Could you check a few things on this model? Use its own coordinates, in mm. Face numbers are marked on the shaded views. A direction names the side the tool comes from. Coordinates: 2 decimals unless noted, no trailing zeros. Order: outer loops, then holes, each group sorted by start corner. A loop starts at its lowest first (then second) coordinate and runs counter-clockwise, first axis right, second up. Notation, with made-up numbers: (-20.5, 30) -> (23.5, 30) arc R29 cw to (23.5, 53) -> close; hole circle Ø6 at (6, 27). An arc over 180 degrees is marked (long way). Use a Markdown table: item, result. Add a question column.
1) Thinking about a two-plate mould opening in X: for the marked faces 4 and 5, which applies, +X half, -X half, draft (parallel to the pull), parting line (faces both ways), or undercut?
2) If I drill on L1, parallel to Y at x = -23, z = -102.5; L2, parallel to X at y = 18, z = -72.5; L3, parallel to Y at x = 32, z = -102, over which ranges is the centre line in solid material (lowest first)? Write a range as [from, to].
3) If we section it at A-A (z = -102.5): Write out the boundary of the cut face in (x, y), plus the area to 3 significant figures.
4) Which directions (+Z, -Z, +X, -X, +Y, -Y) give clear straight access to the entire face, cutting with the end or side of a thin tool? Please do the marked faces 1, 2 and 3.
5) Will these pins go through, and if not, where does the flat tip stop? pin 1 Ø4 at (y, z) = (109, -3) entering from +X; pin 2 Ø12 at (x, y) = (-95, 80.5) entering from +Z; pin 3 Ø12 at (y, z) = (82, 74) entering from -X.
6) If we section it at C-C (x = -82): Write out the boundary of the cut face in (y, z), plus the area to 3 significant figures.
7) If we section it at D-D (z = -47): Write out the boundary of the cut face in (x, y), plus the area to 3 significant figures.
8) If we section it at B-B (y = 59): Write out the boundary of the cut face in (x, z), plus the area to 3 significant figures.
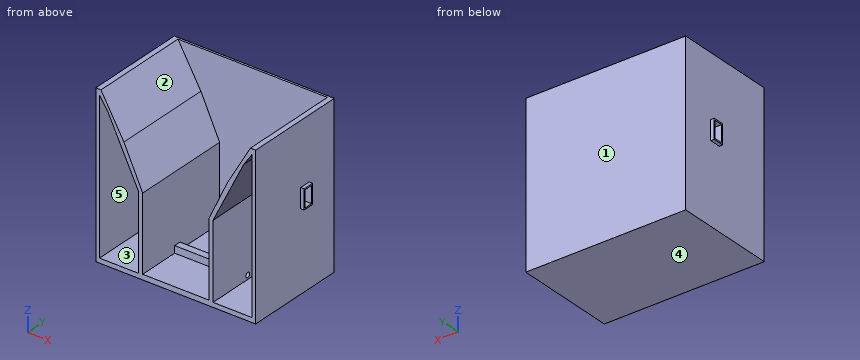
Autodesk Inventor part; units mm, degrees
ref_plane "YZ Plane" through (0, 0, 0) normal (1, 0, 0) x (0, 1, 0)
ref_plane "XZ Plane" through (0, 0, 0) normal (0, 1, 0) x (-1, 0, 0)
ref_plane "XY Plane" through (0, 0, 0) normal (0, 0, 1) x (1, 0, 0)
sketch "Эскиз1" plane through (0, 0, 0) normal (0, 1, 0) x (-1, 0, 0)
  line L0 (-115, -115) -> (115, -115)
  line L1 (115, -115) -> (115, 115)
  line L2 (-115, 115) -> (-115, -115)
  line L3 (-115, -115) -> (115, 115) construction
  line L4 (115, -115) -> (-115, 115) construction
  line L5 (-107.5, -107.5) -> (107.5, -107.5)
  line L6 (107.5, -107.5) -> (107.5, 107.5)
  line L7 (-107.5, 107.5) -> (-107.5, -107.5)
  line L8 (-107.5, -107.5) -> (107.5, 107.5) construction
  line L9 (107.5, -107.5) -> (-107.5, 107.5) construction
  line L10 (107.5, 107.5) -> (107.5, 115)
  line L11 (-107.5, 107.5) -> (-107.5, 115)
  line L12 (115, 115) -> (107.5, 115)
  line L13 (-107.5, 115) -> (-115, 115)
  line L14 (107.5, 115) -> (74.5, 57.8423)
  line L15 (107.5, 115) -> (173.5, 115) construction
  line L16 (74.5, 57.8423) -> (47.5277, 0)
  line L17 (74.5, 57.8423) -> (138.3219, 57.8423) construction
  line L18 (47.5277, 0) -> (47.5277, -107.5)
  line L19 (-107.5, 115) -> (-74.5, 57.8423)
  line L20 (-107.5, 115) -> (-41.5, 115) construction
  line L21 (-74.5, 57.8423) -> (-47.5277, 0)
  line L22 (-74.5, 57.8423) -> (-10.6781, 57.8423) construction
  line L23 (-47.5277, 0) -> (-47.5277, -107.5)
  point P0 (0, 0)
  dimension "d0" = 230
  dimension "d1" = 230
  dimension "d4" = 66
  dimension "d5" = 120
  dimension "d6" = 115
  dimension "d7" = 66
  dimension "d8" = 60
  dimension "d9" = 65
extrude "Выдавливание1" add sketch "Эскиз1" along normal blind 150
sketch "Эскиз2" plane through (0, 150, 0) normal (0, 1, 0) x (1, 0, 0)
  line L0 (97.5879, -89.6233) -> (53.6439, -0.306)
  line L1 (53.6439, -0.306) -> (53.6439, 108.3759)
  line L2 (53.6439, 108.3759) -> (109.6776, 108.3759)
  line L3 (109.6776, 108.3759) -> (109.6776, -107.4647)
  line L4 (109.6776, -107.4647) -> (97.5879, -89.6233)
  line L5 (0, -179.4064) -> (0, 240.0482)
  line L6 (-97.5879, -89.6233) -> (-53.6439, -0.306)
  line L7 (-53.6439, -0.306) -> (-53.6439, 108.3759)
  line L8 (-53.6439, 108.3759) -> (-109.6776, 108.3759)
  line L9 (-109.6776, 108.3759) -> (-109.6776, -107.4647)
  line L10 (-109.6776, -107.4647) -> (-97.5879, -89.6233)
  point P0 (0, 0)
extrude "Выдавливание2" cut sketch "Эскиз2" against normal blind 135161
sketch "Эскиз3" plane through (0, 150, 0) normal (0, 1, 0) x (1, 0, 0)
  line L0 (-107.5, -115) -> (-115, -115)
  line L1 (115, 115) -> (-115, 115)
  line L2 (-115, 115) -> (-115, -115)
  line L3 (-115, -115) -> (115, -115)
  line L4 (115, -115) -> (115, 115)
  line L5 (115, 115) -> (-115, -115) construction
  line L6 (-115, 115) -> (115, -115) construction
  point P0 (0, 0)
extrude "Выдавливание3" add sketch "Эскиз3" against normal blind 3
sketch "Эскиз4" plane through (0, 0, 0) normal (0, -1, 0) x (1, 0, 0)
  line L0 (-115, -115) -> (115, -115)
  line L1 (115, 115) -> (-115, 115)
  line L2 (-115, 115) -> (-115, -115)
  line L3 (-115, -115) -> (115, -115)
  line L4 (115, -115) -> (115, 115)
  line L5 (115, 115) -> (-115, -115) construction
  line L6 (-115, 115) -> (115, -115) construction
  point P0 (0, 0)
  dimension "d16" = 230
  dimension "d17" = 230
extrude "Выдавливание4" cut sketch "Эскиз4" against normal blind 3
sketch "Эскиз5" plane through (-47.5277, 147, -107.5) normal (0, 0, 1) x (1, 0, 0)
  line L0 (95.0554, -144) -> (95.0554, 0)
  line L1 (-0.0319, -84.1415) -> (95.0554, -84.1415)
  line L2 (95.0554, -84.1415) -> (95.0554, -74.1415)
  line L3 (95.0554, -74.1415) -> (-0.0319, -74.1415)
  line L4 (-0.0319, -74.1415) -> (-0.0319, -84.1415)
  point P0 (47.5277, -147)
  dimension "d20" = 10
extrude "Выдавливание5" add sketch "Эскиз5" along normal blind 10
sketch "Эскиз6" plane through (53.6439, 147, 0.306) normal (1, 0, 0) x (0, 0, -1)
  line L0 (107.806, -74.1415) -> (97.806, -74.1415)
  line L1 (97.806, -74.1415) -> (97.806, -84.1415)
  line L2 (97.806, -84.1415) -> (107.806, -84.1415)
  line L3 (107.806, -144) -> (107.806, -84.1415)
  line L4 (107.806, -144) -> (0.306, -144)
  line L5 (0.306, -144) -> (0.306, 0)
  line L6 (0.306, 0) -> (107.806, 0)
  line L7 (107.806, -74.1415) -> (107.806, 0)
  circle A0 centre (102.806, -79.1415) radius 3.5
  point P0 (0.306, -147)
  dimension "d23" = 7
extrude "Выдавливание6" cut sketch "Эскиз6" against normal blind 113.25 contours A0
sketch "Эскиз7" plane through (115, 150, 115) normal (1, 0, 0) x (0, 0, -1)
  line L0 (114.694, -3) -> (114.694, -147)
  line L1 (114.694, -60.802) -> (90.694, -60.802)
  line L2 (90.694, -60.802) -> (90.694, -48.802)
  line L3 (90.694, -48.802) -> (114.694, -48.802)
  line L4 (114.694, -48.802) -> (114.694, -60.802)
  line L5 (116.694, -62.802) -> (88.694, -62.802)
  line L6 (88.694, -62.802) -> (88.694, -46.802)
  line L7 (88.694, -46.802) -> (116.694, -46.802)
  line L8 (116.694, -46.802) -> (116.694, -62.802)
  line L9 (116.694, -62.802) -> (88.694, -46.802) construction
  line L10 (88.694, -62.802) -> (116.694, -46.802) construction
  point P0 (115, -150)
  point P1 (102.694, -54.802)
  point P2 (114.694, -48.802)
  dimension "d26" = 24
  dimension "d27" = 12
  dimension "d28" = 28
  dimension "d29" = 16
extrude "Выдавливание7" add sketch "Эскиз7" along normal blind 5 contours L0 L7 L8 L5 | L3 L2 L1 L0 L5 L6 L7
extrude "Выдавливание8" cut sketch "Эскиз7" against normal blind 44.75 contours L0 L1 L2 L3
pattern_linear "Прямоуг.массив1" count 2 spacing 235 along (-1, 0, 0) of "Выдавливание7"
sketch "Эскиз8" plane through (-115, 89.198, 0.306) normal (-1, 0, 0) x (0, 0, 1)
  line L0 (24, 12) -> (24, 0)
  line L1 (24, 12) -> (0, 12)
  line L2 (24, 0) -> (0, 0)
  line L3 (0, 0) -> (0, 12)
  line L4 (0, 12) -> (24, 12)
  line L5 (24, 12) -> (24, 0)
  point P0 (-0.306, -89.198)
extrude "Выдавливание9" cut sketch "Эскиз8" against normal blind 18
properties part number "qzawsxedcfvgbhnjmk,l."
Answer sheet:
| question | item | result |
|---|---|---|
| 1 | face 4 | draft |
| 1 | face 5 | undercut |
| 2 | L1 | [62.86, 64.36], [71.36, 72.86], [147, 150] |
| 2 | L2 | [-115, -109.68], [-53.64, -47.53], [47.53, 53.64], [109.68, 115] |
| 2 | L3 | [62.86, 64.39], [71.32, 72.86], [147, 150] |
| 3 | outline | (-115, 3) -> (-109.68, 3) -> (-109.68, 147) -> (-53.64, 147) -> (-53.64, 71.36) -> (53.64, 71.36) -> (53.64, 147) -> (109.68, 147) -> (109.68, 3) -> (115, 3) -> (115, 150) -> (-115, 150) -> close; (-53.64, 3) -> (-47.53, 3) -> (-47.53, 62.86) -> (47.53, 62.86) -> (47.53, 3) -> (53.64, 3) -> (53.64, 64.36) -> (-53.64, 64.36) -> close; hole (-47.53, 72.86) -> (47.53, 72.86) -> (47.53, 147) -> (-47.53, 147) -> close |
| 3 | area | 4,180 mm2 |
| 4 | face 1 | +Z, -Z, +X, -X, +Y |
| 4 | face 2 | +Z, -Y |
| 4 | face 3 | -Y |
| 5 | pin 1 | x = 115 |
| 5 | pin 2 | z = 103.74 |
| 5 | pin 3 | x = -115 |
| 6 | outline | (3, -115) -> (150, -115) -> (150, 115) -> (147, 115) -> (147, 70.83) -> (3, 70.83) -> (3, 57.94) -> (147, 57.94) -> (147, -108.38) -> (3, -108.38) -> close |
| 6 | area | 3,500 mm2 |
| 7 | outline | (-115, 3) -> (-109.68, 3) -> (-109.68, 147) -> (-53.64, 147) -> (-53.64, 3) -> (-47.53, 3) -> (-47.53, 147) -> (47.53, 147) -> (47.53, 3) -> (53.64, 3) -> (53.64, 147) -> (109.68, 147) -> (109.68, 3) -> (115, 3) -> (115, 150) -> (-115, 150) -> close |
| 7 | area | 3,980 mm2 |
| 8 | outline | (-115, -115) -> (115, -115) -> (115, 115) -> (107.5, 115) -> (74.5, 57.84) -> (47.53, 0) -> (47.53, -107.5) -> (-47.53, -107.5) -> (-47.53, 0) -> (-74.5, 57.84) -> (-107.5, 115) -> (-115, 115) -> close; hole (-109.68, -108.38) -> (-53.64, -108.38) -> (-53.64, 0.31) -> (-97.59, 89.62) -> (-109.68, 107.46) -> close; hole (53.64, -108.38) -> (109.68, -108.38) -> (109.68, 107.46) -> (97.59, 89.62) -> (53.64, 0.31) -> close |
| 8 | area | 6,740 mm2 |
